Read the model definition and answer for the solid it produces. Units are mm, in the model's axes. A direction names the side the tool comes from. Round coordinates to 2 decimals unless told otherwise and drop trailing zeros. Write each loop counter-clockwise with the first axis right and the second up, starting at its lowest first coordinate (ties: lowest second). Pieces come first, ordered by that corner, then holes. Notation, with made-up numbers: (58, 27) - (109, 27) arc R19 ccw to (109, 37) - close; hole circle Ø10 at (-30, -3.5). An arc over 180 degrees is marked (long way). One line per item, written item: value. Start each with the question number.
(1) A cutting plane is placed at C-C, the plane y = 48. Determine the outline of the cut face in (x, z) (3 decimals), plus the area to 3 significant figures.
(2) For faces 4 (the face through (2, 0, 15)), 5 (the face through (2, 48, 30)), 6 (the face through (2, 65, 15)), determine the directions among +Z, -Z, +X, -X, +Y, -Y from which every point of the face is accessible in a straight line to the end or side of a thin tool.
(3) A cutting plane is placed at D-D, the plane z = 6. Determine the outline of the cut face in (x, y), plus the area to 3 significant figures.
(4) Flat-ended cylindrical pins translate along their axes: pin 1 Ø1.4 at (x, z) = (1, -12.5) entering from +Y; pin 2 Ø2.5 at (x, y) = (2, 46.5) entering from +Z; pin 3 Ø5 at (y, z) = (18, 23) entering from -X; pin 4 Ø1.4 at (x, y) = (2.5, 43.5) entering from -Z. Find the tip coordinate at first contact, or state that the pin passes through.
(5) A cutting plane is placed at A-A, the plane y = 78. Determine the outline of the cut face in (x, z) (3 decimals), plus the area to 3 significant figures.
(6) A cutting plane is placed at B-B, the plane x = 1.3. Determine the outline of the cut face in (y, z) (3 decimals), plus the area to 3 significant figures.
(7) The mould has two halves that part along Z. Classify faces 1 (the face through (2.41, 51.1, 6.31)), 2 (the face through (2.347, 87.719, 2.406)), 3 (the face through (2, 6, -12)): +Z half, -Z half, draft (parallel to the pull), parting line (faces both ways), or undercut.
(8) Find the intervals of material crossed by L1, parallel to Z at x = 2.4, y = 42.5; L2, parallel to Y at x = 0.9, z = 16; L3, parallel to Y at x = 3.55, z = 8, in increasing order.
from build123d import *

# Parameters (mm, degrees)
RESSALTO_EXTRUS_O1_DEPTH   = 30
ESBO_O2_W                  = 12
ESBO_O2_H                  = 94
CORTE_EXTRUS_O1_DEPTH      = 118.541482039
ESBO_O3_W                  = 30
ESBO_O3_H                  = 10
CORTE_EXTRUS_O2_DEPTH      = 118.541482039
ESBO_O4_W                  = 3.6
ESBO_O4_H                  = 30
CORTE_EXTRUS_O3_DEPTH      = 108.498837203
ESBO_O5_W                  = 56.4
ESBO_O5_H                  = 6
RESSALTO_EXTRUS_O2_DEPTH   = 16
ESBO_O6_W                  = 56.4
ESBO_O6_H                  = 6
RESSALTO_EXTRUS_O3_DEPTH   = 16
FILETE1_R                  = 8
FILETE2_R                  = 8
FILETE3_R                  = 8
FILETE4_R                  = 4
ESBO_O7_R                  = 3.175
CORTE_EXTRUS_O4_DEPTH      = 113.943171551
ESBO_O8_R                  = 3.25
CORTE_EXTRUS_O5_DEPTH      = 112.143870726
CORTE_EXTRUS_O6_DEPTH      = 113.943171551
CORTE_EXTRUS_O6_DEPTH_BACK = 1.24
ESBO_O9_W                  = 62
ESBO_O9_H                  = 90
ESBO_O10_W                 = 4.76
ESBO_O10_H                 = 130
CORTE_EXTRUS_O7_DEPTH      = 102.186252031
ESBO_O11_W                 = 4.76
ESBO_O11_H                 = 30
RESSALTO_EXTRUS_O4_DEPTH   = 4.76


with BuildPart() as part:
    # Esboço1 → Ressalto-extrusão1 (new body)
    with BuildSketch(Plane.XY):
        Polygon((0, 0), (0, 100), (60, 0), align=None)
    extrude(amount=RESSALTO_EXTRUS_O1_DEPTH)

    # Esboço2 → Corte-extrusão1 (cut, through all)
    with BuildSketch(Plane.ZY.offset(-6)):
        with Locations((24, 53)):
            Rectangle(ESBO_O2_W, ESBO_O2_H)
        with Locations((6, 53)):
            Rectangle(ESBO_O2_W, ESBO_O2_H)
    extrude(amount=-CORTE_EXTRUS_O1_DEPTH, mode=Mode.SUBTRACT)

    # Esboço3 → Corte-extrusão2 (cut, through all)
    with BuildSketch(Plane(origin=(6, 0, 0), x_dir=(0, 0, -1), z_dir=(1, 0, 0))):
        with Locations((-15, 95)):
            Rectangle(ESBO_O3_W, ESBO_O3_H)
    extrude(amount=-CORTE_EXTRUS_O2_DEPTH, mode=Mode.SUBTRACT)

    # Esboço4 → Corte-extrusão3 (cut, through all)
    with BuildSketch(Plane(origin=(0, 6, 0), x_dir=(1, 0, 0), z_dir=(0, 1, 0))):
        with Locations((58.2, -15)):
            Rectangle(ESBO_O4_W, ESBO_O4_H)
    extrude(amount=-CORTE_EXTRUS_O3_DEPTH, mode=Mode.SUBTRACT)

    # Esboço5 → Ressalto-extrusão2 (add)
    with BuildSketch(Plane.XY.offset(30)):
        with Locations((28.2, 3)):
            Rectangle(ESBO_O5_W, ESBO_O5_H)
    extrude(amount=RESSALTO_EXTRUS_O2_DEPTH)

    # Esboço6 → Ressalto-extrusão3 (add)
    with BuildSketch(Plane(origin=(0, 0, 0), x_dir=(-1, 0, 0), z_dir=(0, 0, -1))):
        with Locations((-28.2, 3)):
            Rectangle(ESBO_O6_W, ESBO_O6_H)
    extrude(amount=RESSALTO_EXTRUS_O3_DEPTH)

    # Filete1
    filete1_edges = [part.edges().sort_by_distance(p)[0] for p in [
        (3, 6, 0),
        (3, 6, 30),
    ]]
    fillet(filete1_edges, radius=FILETE1_R)

    # Filete2
    filete2_edges = [part.edges().sort_by_distance(p)[0] for p in [
        (56.4, 3, -16),
        (56.4, 3, 46),
    ]]
    fillet(filete2_edges, radius=FILETE2_R)

    # Filete3
    filete3_edges = [part.edges().sort_by_distance(p)[0] for p in [
        (3, 90, 30),
        (3, 90, 0),
    ]]
    fillet(filete3_edges, radius=FILETE3_R)

    # Filete4
    filete4_edges = [part.edges().sort_by_distance(p)[0] for p in [
        (31.2, 6, 18),
        (31.2, 6, 12),
    ]]
    fillet(filete4_edges, radius=FILETE4_R)

    # Esboço7 → Corte-extrusão4 (cut, through all)
    with BuildSketch(Plane(origin=(6, 0, 0), x_dir=(0, 0, -1), z_dir=(1, 0, 0))):
        with Locations((-23, 78)):
            Circle(ESBO_O7_R)
        with Locations((-23, 48)):
            Circle(ESBO_O7_R)
        with Locations((-23, 18)):
            Circle(ESBO_O7_R)
        with Locations(Location((-7, 18, 0), (0, 0, 180))):
            Circle(ESBO_O7_R)
        with Locations(Location((-7, 48, 0), (0, 0, 180))):
            Circle(ESBO_O7_R)
        with Locations(Location((-7, 78, 0), (0, 0, 180))):
            Circle(ESBO_O7_R)
    extrude(amount=-CORTE_EXTRUS_O4_DEPTH, mode=Mode.SUBTRACT)

    # Esboço8 → Corte-extrusão5 (cut, through all)
    with BuildSketch(Plane(origin=(0, 6, 0), x_dir=(1, 0, 0), z_dir=(0, 1, 0))):
        with Locations(Location((48.4, 8, 0), (0, 0, 270))):
            Circle(ESBO_O8_R)
        with Locations(Location((48.4, -38, 0), (0, 0, 270))):
            Circle(ESBO_O8_R)
        with Locations(Location((16.4, -38, 0), (0, 0, 270))):
            Circle(ESBO_O8_R)
        with Locations(Location((16.4, 8, 0), (0, 0, 270))):
            Circle(ESBO_O8_R)
    extrude(amount=-CORTE_EXTRUS_O5_DEPTH, mode=Mode.SUBTRACT)

    # Esboço9 → Corte-extrusão6 (cut, two sides: drawn at the far end of the back side and taken through both)
    with BuildSketch(Plane(origin=(6, 0, 0), x_dir=(0, 0, -1), z_dir=(1, 0, 0)).offset(-CORTE_EXTRUS_O6_DEPTH_BACK)):
        with Locations((-15, 45)):
            Rectangle(ESBO_O9_W, ESBO_O9_H)
    extrude(amount=CORTE_EXTRUS_O6_DEPTH + CORTE_EXTRUS_O6_DEPTH_BACK, mode=Mode.SUBTRACT)

    # Esboço10 → Corte-extrusão7 (cut, through all)
    with BuildSketch(Plane.ZY):
        with Locations((15, 0)):
            Rectangle(ESBO_O10_W, ESBO_O10_H)
    extrude(amount=-CORTE_EXTRUS_O7_DEPTH, mode=Mode.SUBTRACT)

    # Esboço11 → Ressalto-extrusão4 (add, through all)
    with BuildSketch(Plane.ZY):
        with Locations((15, 15)):
            Rectangle(ESBO_O11_W, ESBO_O11_H)
    extrude(amount=-RESSALTO_EXTRUS_O4_DEPTH)


solid = part.part
Here are the results:
1. outline: (0, 0) - (4.76, 0) - (4.76, 3.825) - (0, 3.825) - close; (0, 10.175) - (4.76, 10.175) - (4.76, 12.62) - (0, 12.62) - close; (0, 17.38) - (4.76, 17.38) - (4.76, 19.825) - (0, 19.825) - close; (0, 26.175) - (4.76, 26.175) - (4.76, 30) - (0, 30) - close
1. area: 59.7 mm²
2. face 4: +Z, -Z, +X, -X, -Y
2. face 5: +Z, +X, -X, +Y
2. face 6: +X, -X
3. outline: (0, 0) - (4.76, 0) - (4.76, 14.99) - (0, 14.99) - close; (0, 21.01) - (4.76, 21.01) - (4.76, 44.99) - (0, 44.99) - close; (0, 51.01) - (4.76, 51.01) - (4.76, 74.99) - (0, 74.99) - close; (0, 81.01) - (4.76, 81.01) - (4.76, 89.75) - (0, 89.75) - close
3. area: 341 mm²
4. pin 1: y = 6
4. pin 2: z = 30
4. pin 3: through
4. pin 4: z = 0
5. outline: (0, 0) - (4.76, 0) - (4.76, 3.825) - (0, 3.825) - close; (0, 10.175) - (4.76, 10.175) - (4.76, 19.825) - (0, 19.825) - close; (0, 26.175) - (4.76, 26.175) - (4.76, 30) - (0, 30) - close
5. area: 82.3 mm²
6. outline: (0, -16) - (6, -16) - (6, -8) arc R8 cw to (14, 0) - (82, 0) arc R8 ccw to (90, 8) - (90, 22) arc R8 ccw to (82, 30) - (14, 30) arc R8 cw to (6, 38) - (6, 46) - (0, 46) - close; hole circle Ø6.35 at (18, 7); hole circle Ø6.35 at (18, 23); hole (30, 12.62) - (65, 12.62) - (65, 17.38) - (30, 17.38) - close; hole circle Ø6.35 at (48, 7); hole circle Ø6.35 at (48, 23); hole circle Ø6.35 at (78, 7); hole circle Ø6.35 at (78, 23)
6. area: 2,540 mm²
7. face 1: undercut
7. face 2: -Z half
7. face 3: draft
8. L1: 0 to 12.62, 17.38 to 30
8. L2: 0 to 30, 65 to 90
8. L3: 0 to 14.99, 21.01 to 44.99, 51.01 to 74.99, 81.01 to 90
